Verification items for this drawing (mm, ordinates from the low corner). A direction names the side the tool comes from. Give positions to 0.01 mm unless a question says otherwise; leave off trailing zeros. Loops run counter-clockwise (first coordinate to the right, second up) from the corner with the lowest first, then second, coordinate; pieces in that order, holes last. Notation, with made-up numbers: M 34.25,-38 L 85.25,-38 A32 cw 85.25,-4 Z; hole C 1,80.5 d4. An arc over 180 degrees is marked long. Use a Markdown table: item, result.
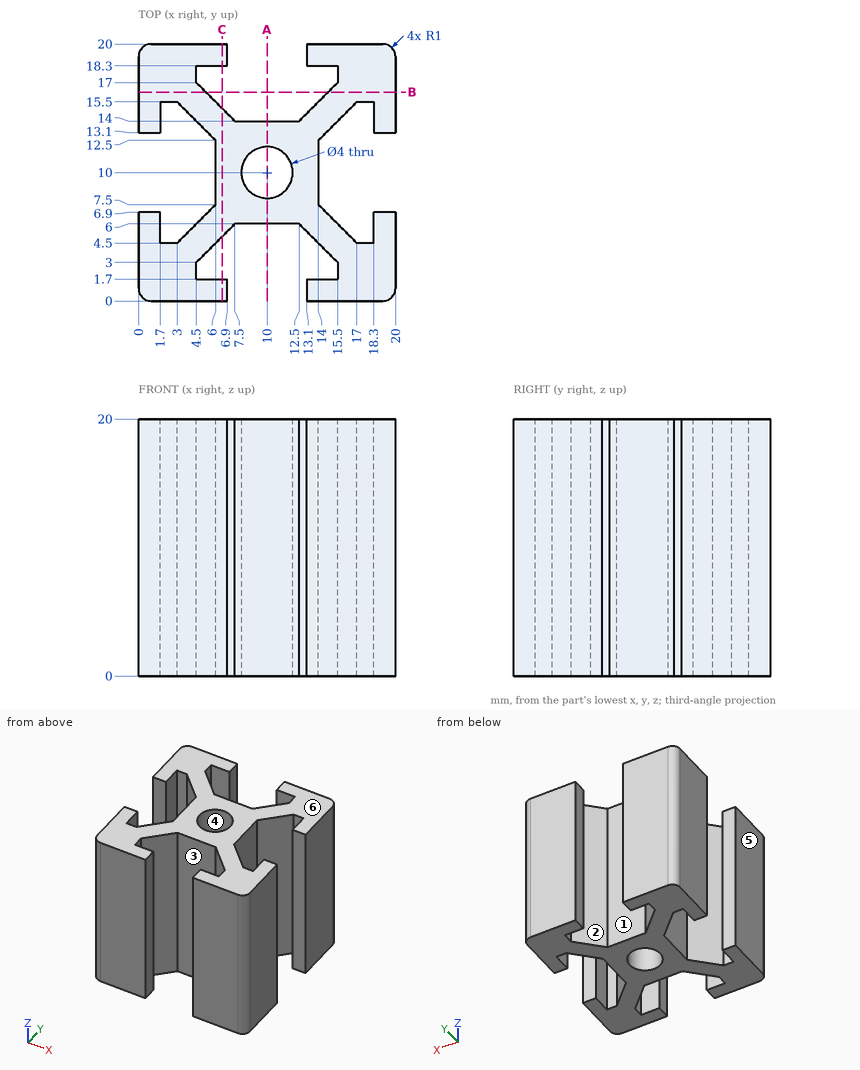
(1) Cross-section at B-B on y = 16.25. Record the cut outline in (x, z), then the cut area to 3 significant figures.
Results below:
| item | result |
|---|---|
| outline | M 0,0 L 5.25,0 L 5.25,20 L 0,20 Z; M 14.75,0 L 20,0 L 20,20 L 14.75,20 Z |
| area | 210 mm^2 |
(2) Draft check along X on the marked faces 4, 5 and 6. Enter one of: +X half, -X half, draft (parallel to the pull), parting line (faces both ways), or undercut.
Results below:
| item | result |
|---|---|
| face 4 | undercut |
| face 5 | -X half |
| face 6 | draft |
(3) Cross-section at A-A on x = 10. Record the cut outline in (y, z).
Results below:
| item | result |
|---|---|
| outline | M 6,0 L 8,0 L 8,20 L 6,20 Z; M 12,0 L 14,0 L 14,20 L 12,20 Z |
(4) Cross-section at C-C on x = 6.5. Record the cut outline in (y, z), then the cut area to 3 significant figures.
Results below:
| item | result |
|---|---|
| outline | M 0,0 L 1.7,0 L 1.7,20 L 0,20 Z; M 5,0 L 15,0 L 15,20 L 5,20 Z; M 18.3,0 L 20,0 L 20,20 L 18.3,20 Z |
| area | 268 mm^2 |
(5) Material ranges on line 1 (Y direction, x = 10, z = 12.25); line 2 (Y direction, x = 13.5, z = 11.5); line 3 (Y direction, x = 18.5, z = 16.5), recorded low to high.
Results below:
| item | result |
|---|---|
| line 1 | 6 to 8, 12 to 14 |
| line 2 | 0 to 1.7, 5 to 15, 18.3 to 20 |
| line 3 | 0 to 6.9, 13.1 to 20 |
(6) Gauge pin test, flat ends, axial feed: P1, Ø4, axis at x = 8, z = 12.5, coming from the +Y side; P2, Ø4, axis at y = 10, z = 11, coming from the -X side. Record the tip position at first contact, or that the pin passes through.
Results below:
| item | result |
|---|---|
| P1 | y = 20 |
| P2 | x = 6 |
(7) Set-up check for the marked faces 1, 2 and 3: record each of +Z, -Z, +X, -X, +Y, -Y from which the full face is reachable in a straight line by a thin tool's end or side.
Results below:
| item | result |
|---|---|
| face 1 | +Z, -Z, +Y |
| face 2 | +Z, -Z |
| face 3 | +Z, -Z, -Y |
